Autodesk Inventor part; units mm, degrees
ref_plane "YZ Plane" through (0, 0, 0) normal (1, 0, 0) x (0, 1, 0)
ref_plane "XZ Plane" through (0, 0, 0) normal (0, 1, 0) x (-1, 0, 0)
ref_plane "XY Plane" through (0, 0, 0) normal (0, 0, 1) x (1, 0, 0)
sketch "Sketch1" plane through (0, 0, 0) normal (0, 1, 0) x (-1, 0, 0)
  line L0 (-9.45, 13.9) -> (9.45, 13.9)
  line L1 (9.45, 13.9) -> (9.45, 12.4)
  line L2 (9.45, 12.4) -> (-9.45, 12.4)
  line L3 (-9.45, 12.4) -> (-9.45, 13.9)
  line L4 (9.45, 12.4) -> (6.45, 12.4)
  line L5 (6.45, 12.4) -> (6.45, -9)
  line L6 (6.45, -9) -> (9.45, -9)
  line L7 (9.45, -9) -> (9.45, 12.4)
  line L8 (-9.45, 12.4) -> (-7.95, 12.4)
  line L9 (-7.95, 12.4) -> (-7.95, -9)
  line L10 (-7.95, -9) -> (-9.45, -9)
  line L11 (-9.45, -9) -> (-9.45, 12.4)
  line L12 (-7.95, -9) -> (-9.45, -9)
  line L13 (-9.45, -9) -> (-9.45, -12)
  line L14 (-9.45, -12) -> (-7.95, -12)
  line L15 (-7.95, -12) -> (-7.95, -9)
  line L16 (1.45, -9) -> (9.45, -9)
  line L17 (9.45, -9) -> (9.45, -12)
  line L18 (9.45, -12) -> (1.45, -12)
  line L19 (1.45, -12) -> (1.45, -9)
  line L20 (-9.45, -12) -> (-7.95, -12)
  line L21 (9.45, -12) -> (6.45, -12)
  line L22 (-7.95, -12) -> (-4.95, -12)
  line L23 (-4.95, -12) -> (-4.95, -9)
  line L24 (-4.95, -9) -> (-7.95, -9)
  line L25 (-7.95, -9) -> (-7.95, -12)
  point P0 (0, 0)
  point P1 (0, 12.4)
  dimension "d0" = 1.5
  dimension "d1" = 3
  dimension "d2" = 1.5
  dimension "d3" = 3
  dimension "d4" = 3
  dimension "d5" = 0
  dimension "d6" = 5
  dimension "d7" = 14.4
  dimension "d8" = 21.4
  dimension "d9" = 21.4
  dimension "d12" = 0
  dimension "d13" = 0
  dimension "d38" = 3
extrude "Extrusion1" add sketch "Sketch1" along normal blind 10 contours L0 L1 L2 L3 | L7 L6 L5 L2 | L17 L18 L19 L16 L6
sketch "Sketch8" plane through (0, 0, 0) normal (0, -1, 0) x (1, 0, 0)
  line L0 (2.9056, 13.9) -> (14.45, 13.9)
  line L1 (14.45, 13.9) -> (14.45, -22.6)
  line L2 (14.45, -22.6) -> (2.9056, -22.6)
  line L3 (2.9056, -22.6) -> (2.9056, 13.9)
  line L4 (-9.45, 13.9) -> (9.45, 13.9)
  point P0 (0, 0)
extrude "Extrusion6" cut sketch "Sketch8" against normal blind 5
sketch "Sketch9" plane through (0, 0, 0) normal (0, -1, 0) x (1, 0, 0)
  line L0 (2.9056, 12.4) -> (2.9056, 13.9)
  line L1 (-9.45, 13.9) -> (2.9056, 13.9)
  line L2 (-9.45, 13.9) -> (-9.45, -12)
  line L3 (-9.45, -12) -> (-1.45, -12)
  line L4 (-1.45, -12) -> (-1.45, -9)
  line L5 (-1.45, -9) -> (-6.45, -9)
  line L6 (-6.45, 12.4) -> (-6.45, -9)
  line L7 (2.9056, 12.4) -> (-6.45, 12.4)
  line L8 (-6.45, -9) -> (-1.45, -9)
  line L9 (-9.45, -12) -> (-9.45, 13.9)
  line L10 (-6.45, -9) -> (-9.45, -9)
  line L11 (-9.45, -9) -> (-9.45, 12.4)
  line L12 (-9.45, 12.4) -> (-6.45, 12.4)
  line L13 (-6.45, 12.4) -> (-6.45, -9)
  point P0 (0, 0)
extrude "Extrusion7" add sketch "Sketch9" along normal blind 17.5 contours L6 L10 L2 L12
sketch "Sketch10" plane through (-9.45, 0, 13.9) normal (-1, 0, 0) x (0, 0, 1)
  line L0 (-22.9, -17.5) -> (-1.5, -17.5)
  line L1 (-1.5, 0) -> (-1.5, -17.5)
  line L2 (-22.9, -17.5) -> (-1.5, -17.5)
  line L3 (-1.5, -17.5) -> (-1.5, -14.5)
  line L4 (-1.5, -14.5) -> (-22.9, -14.5)
  line L5 (-22.9, -14.5) -> (-22.9, -17.5)
  point P0 (-13.9, 0)
  dimension "d41" = 3
extrude "Extrusion8" add sketch "Sketch10" along normal blind 6
sketch "Sketch11" plane through (-9.45, -14.5, 12.4) normal (0, 1, 0) x (1, 0, 0)
  line L0 (0, 21.4) -> (0, 0)
  line L1 (0, 21.4) -> (-6, 21.4)
  line L2 (-6, 0) -> (-6, 21.4)
  line L3 (0, 0) -> (-6, 0)
  line L4 (3, 21.4) -> (-6, 21.4)
  line L5 (-3, 21.4) -> (-3, 0) construction
  circle A0 centre (-3, 4.7) radius 2.25
  circle A1 centre (-3, 16.7) radius 2.25
  line L6 (-6, 0) -> (-6, 21.4)
  line L7 (-6, 10.7) -> (0, 10.7) construction
  point P0 (9.45, 12.4)
  dimension "d44" = 4.5
  dimension "d45" = 4.5
  dimension "d50" = 6
  dimension "d51" = 6
extrude "Extrusion9" cut sketch "Sketch11" against normal blind 3 contours A0 | A1
sketch "Sketch12" plane through (0, 0, 0) normal (0, -1, 0) x (1, 0, 0)
  line L0 (-9.45, 12.4) -> (-6.45, 12.4)
  line L1 (2.9056, 12.4) -> (-6.45, 12.4)
  line L2 (2.9056, 12.4) -> (2.9056, 13.9)
  line L3 (-9.45, 13.9) -> (2.9056, 13.9)
  line L4 (-9.45, 13.9) -> (-9.45, 12.4)
  point P0 (0, 0)
extrude "Extrusion10" add sketch "Sketch12" along normal blind 17.5
sketch "Sketch13" plane through (-9.45, 10, 13.9) normal (0, 0, 1) x (1, 0, 0)
  line L0 (12.3556, -27.5) -> (12.3556, -5)
  line L1 (12.3556, -5) -> (18.9, -5)
  line L2 (18.9, -5) -> (18.9, 0)
  line L3 (0, 0) -> (18.9, 0)
  line L4 (0, -27.5) -> (0, 0)
  line L5 (12.3556, -27.5) -> (0, -27.5)
  line L6 (12.3556, -5) -> (12.3556, -27.5)
  line L7 (0, -27.5) -> (0, 0)
  line L8 (12.3556, -27.5) -> (0, -27.5)
  line L9 (0, -27.5) -> (0, -24.5)
  line L10 (0, -24.5) -> (12.3556, -24.5)
  line L11 (12.3556, -24.5) -> (12.3556, -27.5)
  point P0 (9.45, -10)
  dimension "d54" = 3
extrude "Extrusion11" add sketch "Sketch13" along normal blind 10 contours L5 L4 L10 L0
sketch "Sketch14" plane through (-9.45, -14.5, 13.9) normal (0, 1, 0) x (1, 0, 0)
  line L0 (0, 0) -> (12.3556, 0)
  line L1 (0, 0) -> (0, -10)
  line L2 (12.3556, -10) -> (0, -10)
  line L3 (12.3556, 0) -> (12.3556, -10)
  circle A0 centre (6.1778, -5) radius 2.25
  point P0 (9.45, 13.9)
  dimension "d57" = 4.5
extrude "Extrusion12" cut sketch "Sketch14" against normal blind 3 contours A0
sketch "Sketch15" plane through (-9.45, 0, -12) normal (-1, 0, 0) x (0, 0, 1)
  line L0 (3, -14.5) -> (24.4, -14.5)
  line L1 (24.4, -17.5) -> (24.4, -14.5)
  line L2 (24.4, -17.5) -> (35.9, -17.5)
  line L3 (35.9, -14.5) -> (35.9, -17.5)
  line L4 (25.9, -14.5) -> (35.9, -14.5)
  line L5 (25.9, -14.5) -> (25.9, 10)
  line L6 (0, 10) -> (25.9, 10)
  line L7 (0, 0) -> (0, 10)
  line L8 (3, 0) -> (0, 0)
  line L9 (3, 0) -> (3, -14.5)
  line L10 (24.4, -17.5) -> (35.9, -17.5)
  line L11 (24.4, -17.5) -> (24.4, -14.5)
  line L12 (35.9, -17.5) -> (24.4, -17.5)
  line L13 (24.4, -17.5) -> (24.4, -14.5)
  line L14 (24.4, -14.5) -> (35.9, -14.5)
  line L15 (35.9, -14.5) -> (35.9, -17.5)
  point P0 (12, 0)
extrude "Extrusion13" add sketch "Sketch15" along normal blind 6 contours L14 L4 L3 L2 L1
sketch "Sketch16" plane through (0, -17.5, 0) normal (0, -1, 0) x (1, 0, 0)
  circle A0 centre (-3.2722, 18.9) radius 2.25
  circle A1 centre (-12.45, 7.7) radius 2.25
  circle A2 centre (-12.45, -4.3) radius 2.25
  line L0 (-6.45, -9) -> (-15.45, -9)
  line L1 (-6.45, -9) -> (-6.45, 12.4)
  line L2 (-6.45, 12.4) -> (2.9056, 12.4)
  line L3 (2.9056, 12.4) -> (2.9056, 23.9)
  line L4 (2.9056, 23.9) -> (-15.45, 23.9)
  line L5 (-15.45, -9) -> (-15.45, 23.9)
  point P0 (0, 0)
equation "\"sp\" = 0.4"
properties part number "MotorMount"
The listing builds one solid part. Answer for the finished solid, in the listing's coordinates (mm). A direction names the side the tool comes from. Round coordinates to 2 decimals unless told otherwise and drop trailing zeros. Loops run counter-clockwise (first coordinate to the right, second up) from the corner with the lowest first, then second, coordinate; pieces in that order, holes last. Notation, with made-up numbers: (8, 62.25) - (49, 62.25) arc R12 cw to (49, 74.25) - close; hole circle Ø4 at (84, 77.25). An arc over 180 degrees is marked (long way). Return JSON: item names as keys, results as strings. Group by question number.
1. Which of the six approach directions +Z, -Z, +X, -X, +Y, -Y give full straight-line access (tool end or side, diameter ignored) to faces 5 (the flat face through (6, 5, 13)), 6 (the flat face through (0, -1, 12.4)), 7 (the flat face through (-9.45, -2, 1)), 8 (the flat face through (-1.45, 5, -11)), 9 (the flat face through (-9, -11, -9))?
2. The part is cut by section A-A on z = -4.3. Determine the outline of the cut face in (x, y).
3. Consider probe 1 along Z at (x, y) = (-12.45, -15.45); probe 2 along Z at (x, y) = (-13.5, -14.75); probe 3 along X at (y, z) = (-15.9, 18.9). Determine where each line is inside the solid, lowest interval first.
4. The part is cut by section D-D on x = -7.5. Determine the outline of the cut face in (y, z).
5. The part is cut by section B-B on x = -12.45. Determine the outline of the cut face in (y, z), then the cut area to 3 significant figures.
6. The mould has two halves that part along X. Classify faces 1 (the cylindrical face through (-10.304, -15.979, 7.024)), 2 (the cylindrical face through (-3.57, -15.98, 16.67)), 3 (the flat face through (-6, -16, 23.9)), 4 (the flat face through (9.45, 7, 13)): pulls with the +X half, pulls with the -X half, needs draft (parallel to the pull), parting line crosses it, or undercut.
7. The part is cut by section C-C on y = -15.75. Determine the outline of the cut face in (x, z).
8. Each of these flat-tipped pins is pushed along its axis until it touches: P1, Ø8, axis at y = -2.5, z = 17.5, coming from the -X side; P2, Ø6, axis at x = -2.5, y = 1, coming from the +Z side; P3, Ø10.5, axis at y = -4, z = 3, coming from the +X side. Where does it stop, or does it pass through?
Resolved:
{
 "1": {"face 5": "+Z, -Z, +X, -Y", "face 6": "+X, +Y, -Y", "face 7": "+Z, -Z, -X, +Y", "face 8": "-Z, +X, +Y, -Y", "face 9": "-Z, +X, -X, -Y"},
 "2": {"outline": "(-15.45, -17.5) - (-14.7, -17.5) - (-14.7, -14.5) - (-15.45, -14.5) - close; (-10.2, -17.5) - (-6.45, -17.5) - (-6.45, 10) - (-9.45, 10) - (-9.45, -14.5) - (-10.2, -14.5) - close"},
 "3": {"probe 1": "z = -9 to -6.55, -2.05 to 5.45, 9.95 to 23.9", "probe 2": "z = -9 to -6.29, -2.31 to 5.71, 9.69 to 23.9", "probe 3": "x = -15.45 to -5.52, -1.02 to 2.91"},
 "4": {"outline": "(-17.5, -9) - (0, -9) - (0, -12) - (10, -12) - (10, 13.9) - (-14.5, 13.9) - (-14.5, 23.9) - (-17.5, 23.9) - close"},
 "5": {"outline": "(-17.5, -9) - (-14.5, -9) - (-14.5, -6.55) - (-17.5, -6.55) - close; (-17.5, -2.05) - (-14.5, -2.05) - (-14.5, 5.45) - (-17.5, 5.45) - close; (-17.5, 9.95) - (-14.5, 9.95) - (-14.5, 23.9) - (-17.5, 23.9) - close", "area": "71.7 mm²"},
 "6": {"face 1": "undercut", "face 2": "undercut", "face 3": "needs draft", "face 4": "pulls with the +X half"},
 "7": {"outline": "(-15.45, -9) - (-6.45, -9) - (-6.45, 12.4) - (2.91, 12.4) - (2.91, 23.9) - (-15.45, 23.9) - close; hole circle Ø4.5 at (-12.45, -4.3); hole circle Ø4.5 at (-12.45, 7.7); hole circle Ø4.5 at (-3.27, 18.9)"},
 "8": {"P1": "stops at x = -9.45", "P2": "stops at z = 13.9", "P3": "stops at x = -6.45"}
}
